Design review of the part built by this model. Coordinates are the model's own, in mm. A direction names the side the tool comes from. Coordinates: 2 decimals unless noted, no trailing zeros. Write each loop counter-clockwise with the first axis right and the second up, starting at its lowest first coordinate (ties: lowest second). Pieces come first, ordered by that corner, then holes.
Q1. For pin 1 Ø1.9 at (x, y) = (5, 25.5) entering from -Z; pin 2 Ø5 at (x, y) = (-20.5, 15.5) entering from -Z; pin 3 Ø2 at (x, z) = (-23.5, 6) entering from +Y, all flat-tipped, find the tip position at first contact; note any pin that passes through.
Q2. For L1, parallel to Y at x = 8, z = 8; L2, parallel to Y at x = 18, z = 6.5 (3 decimals); L3, parallel to X at y = -3.5, z = -2, list the stretches that pass through material, from the lowest coordinate up.
Q3. For faces 1 (the cylindrical face through (-10.211, -24.914, 3.964)), 2 (the flat face through (0.635, 22, 3)), list the 3-axis set-ups (+Z, -Z, +X, -X, +Y, -Y) from which the entire face can be reached by the end or side of a thin tool; tool diameter is ignored.
Q4. The part is to be moulded in two halves that separate along X. For faces 3 (the flat face through (-15.4, -16.3, 2.8)), 4 (the flat face through (28, 0, 11.176)), say which applies: released by +X, released by -X, zero draft, split by the parting line, or undercut.
Q5. Take a section at A-A, the plane z = -6. Write out the cut boundary in (x, y), plus the area to 3 significant figures.
from build123d import *

# Parameters (mm, degrees)
C3A_CAVITYPRISM_DEPTH  = 11.938
SK_C3_RIBS_W           = 19.05
SK_C3_RIBS_H           = 1.27
SK_C3_RIBS_W_2         = 1.27
SK_C3_RIBS_H_2         = 19.05
C3D_RIBS_DEPTH         = 11.938
C2_SCALLOPS_DEPTH      = 47.436868801
C2_SCALLOPS_DEPTH_BACK = 47.436868801
SK_C2_SCALLOPS_R       = 8.382
SK_C5_RIDGE_W          = 3.0426914
SK_C5_RIDGE_H          = 0.381


with BuildPart() as part:
    # SK_C1_profile → C1_MainRevolve (revolve)
    with BuildSketch(Plane(origin=(0, 0, 0), x_dir=(1, 0, 0), z_dir=(0, 1, 0)), mode=Mode.PRIVATE) as c1_mainrevolve_sk:
        with BuildLine():
            Line((0, 17.272), (15.3929334, 17.272))
            ThreePointArc((15.3929334, 17.272), (15.742617524, 17.13249018), (15.900237204, 16.790586666))
            Line((15.900237204, 16.790586666), (16.620448253, 3.048))
            Line((16.620448253, 3.048), (30.48, 3.048))
            Line((30.48, 3.048), (30.48, -11.176))
            Line((30.48, -11.176), (26.924, -11.176))
            ThreePointArc((26.924, -11.176), (19.874523429, -13.957256168), (12.5108462, -15.748))
            Line((12.5108462, -15.748), (0, -15.748))
            Line((0, -15.748), (0, 17.272))
        make_face()
    revolve(c1_mainrevolve_sk.sketch.rotate(Axis((0, 0, -50.8), (0, 0, 1)), 180), axis=Axis((0, 0, -50.8), (0, 0, 1)))

    # SK_C3_Lci → C3a_CavityPrism (cut)
    with BuildSketch(Plane.XY.offset(-3.048)):
        with BuildLine():
            ThreePointArc((27.769715286, -4.872837874), (28.194, 0), (27.769715286, 4.872837874))
            ThreePointArc((27.769715286, 4.872837874), (23.466540126, 9.720159182), (23.081770695, 16.190537286))
            ThreePointArc((23.081770695, 16.190537286), (19.936168589, 19.936168589), (16.190537286, 23.081770695))
            ThreePointArc((16.190537286, 23.081770695), (9.720159182, 23.466540126), (4.872837874, 27.769715286))
            ThreePointArc((4.872837874, 27.769715286), (0, 28.194), (-4.872837874, 27.769715286))
            ThreePointArc((-4.872837874, 27.769715286), (-9.720159182, 23.466540126), (-16.190537286, 23.081770695))
            ThreePointArc((-16.190537286, 23.081770695), (-19.936168589, 19.936168589), (-23.081770695, 16.190537286))
            ThreePointArc((-23.081770695, 16.190537286), (-23.466540126, 9.720159182), (-27.769715286, 4.872837874))
            ThreePointArc((-27.769715286, 4.872837874), (-28.194, 0), (-27.769715286, -4.872837874))
            ThreePointArc((-27.769715286, -4.872837874), (-23.466540126, -9.720159182), (-23.081770695, -16.190537286))
            ThreePointArc((-23.081770695, -16.190537286), (-19.936168589, -19.936168589), (-16.190537286, -23.081770695))
            ThreePointArc((-16.190537286, -23.081770695), (-9.720159182, -23.466540126), (-4.872837874, -27.769715286))
            ThreePointArc((-4.872837874, -27.769715286), (0, -28.194), (4.872837874, -27.769715286))
            ThreePointArc((4.872837874, -27.769715286), (9.720159182, -23.466540126), (16.190537286, -23.081770695))
            ThreePointArc((16.190537286, -23.081770695), (19.936168589, -19.936168589), (23.081770695, -16.190537286))
            ThreePointArc((23.081770695, -16.190537286), (23.466540126, -9.720159182), (27.769715286, -4.872837874))
        make_face()
    extrude(amount=C3A_CAVITYPRISM_DEPTH, mode=Mode.SUBTRACT)


with BuildPart() as c3a_cavityprism_piece_1:
    # of the separate pieces the step leaves, piece 1, a body of its own (c3a_cavityprism_pieces)
    add(part.part.solids().sort_by_distance((-30.48, 0, -3.048))[0])

    # SK_C3_ceiling → C3b_CeilingRing (revolve)
    with BuildSketch(Plane(origin=(0, 0, 0), x_dir=(1, 0, 0), z_dir=(0, 1, 0)), mode=Mode.PRIVATE) as c3b_ceilingring_sk:
        Polygon((25.654, -6.604), (23.368, -8.89), (30.48, -8.89), (30.48, -6.604), align=None)
    revolve(c3b_ceilingring_sk.sketch.rotate(Axis((0, 0, -50.8), (0, 0, 1)), 180), axis=Axis((0, 0, -50.8), (0, 0, 1)))



with BuildPart() as c3a_cavityprism_piece_2:
    # of the separate pieces the step leaves, piece 2, a body of its own (c3a_cavityprism_pieces)
    add(part.part.solids().sort_by_distance((-15.3929334, 0, -17.272))[0])


with BuildPart() as c3a_cavityprism_piece_1_1:
    add(c3a_cavityprism_piece_1.part)

    add(c3a_cavityprism_piece_2.part)  # C3c_HubUp merges C3a_CavityPrism piece 2
    # SK_C3_hub → C3c_HubUp (revolve)
    with BuildSketch(Plane(origin=(0, 0, 0), x_dir=(1, 0, 0), z_dir=(0, 1, 0)), mode=Mode.PRIVATE) as c3c_hubup_sk:
        Polygon((0, 3.048), (16.620448253, 3.048), (17.246092322, -8.89), (0, -8.89), align=None)
    revolve(c3c_hubup_sk.sketch.rotate(Axis((0, 0, -50.8), (0, 0, 1)), 180), axis=Axis((0, 0, -50.8), (0, 0, 1)))

    # SK_C3_ribs → C3d_Ribs (add)
    with BuildSketch(Plane.XY.offset(-3.048)):
        with Locations((19.685, 0)):
            Rectangle(SK_C3_RIBS_W, SK_C3_RIBS_H)
        Polygon((7.633217703, 6.735192091), (21.103601885, 20.205576272), (20.205576272, 21.103601885), (6.735192091, 7.633217703), align=None)
        with Locations((0, 19.685)):
            Rectangle(SK_C3_RIBS_W_2, SK_C3_RIBS_H_2)
        Polygon((-6.735192091, 7.633217703), (-20.205576272, 21.103601885), (-21.103601885, 20.205576272), (-7.633217703, 6.735192091), align=None)
        with Locations((-19.685, 0)):
            Rectangle(SK_C3_RIBS_W, SK_C3_RIBS_H)
        Polygon((-7.633217703, -6.735192091), (-21.103601885, -20.205576272), (-20.205576272, -21.103601885), (-6.735192091, -7.633217703), align=None)
        with Locations((0, -19.685)):
            Rectangle(SK_C3_RIBS_W_2, SK_C3_RIBS_H_2)
        Polygon((6.735192091, -7.633217703), (20.205576272, -21.103601885), (21.103601885, -20.205576272), (7.633217703, -6.735192091), align=None)
    extrude(amount=C3D_RIBS_DEPTH)

    # SK_C2_scallops → C2_Scallops (cut, two sides: drawn at the far end of the back side and taken through both)
    with BuildSketch(Plane.XY.offset(-C2_SCALLOPS_DEPTH_BACK)):
        with Locations((32.618490775, 13.511021263)):
            Circle(SK_C2_SCALLOPS_R)
        with Locations((13.511021263, 32.618490775)):
            Circle(SK_C2_SCALLOPS_R)
        with Locations((-13.511021263, 32.618490775)):
            Circle(SK_C2_SCALLOPS_R)
        with Locations((-32.618490775, 13.511021263)):
            Circle(SK_C2_SCALLOPS_R)
        with Locations((-32.618490775, -13.511021263)):
            Circle(SK_C2_SCALLOPS_R)
        with Locations((-13.511021263, -32.618490775)):
            Circle(SK_C2_SCALLOPS_R)
        with Locations((13.511021263, -32.618490775)):
            Circle(SK_C2_SCALLOPS_R)
        with Locations((32.618490775, -13.511021263)):
            Circle(SK_C2_SCALLOPS_R)
    extrude(amount=C2_SCALLOPS_DEPTH + C2_SCALLOPS_DEPTH_BACK, mode=Mode.SUBTRACT)

    # SK_C4_bore → C4_Bore (revolve, cut)
    with BuildSketch(Plane(origin=(0, 0, 0), x_dir=(1, 0, 0), z_dir=(0, 1, 0)), mode=Mode.PRIVATE) as c4_bore_sk:
        with BuildLine():
            Line((0, 18.542), (6.746875, 18.542))
            Line((6.746875, 18.542), (6.746875, 4.572))
            Line((6.746875, 4.572), (9.144, 4.572))
            Line((9.144, 4.572), (10.1900228, -15.386939))
            ThreePointArc((10.1900228, -15.386939), (10.308227792, -15.643369045), (10.5704894, -15.748))
            Line((10.5704894, -15.748), (10.5704894, -18.288))
            Line((10.5704894, -18.288), (0, -18.288))
            Line((0, -18.288), (0, 18.542))
        make_face()
    revolve(c4_bore_sk.sketch.rotate(Axis((0, 0, -50.8), (0, 0, 1)), 180), axis=Axis((0, 0, -50.8), (0, 0, 1)), mode=Mode.SUBTRACT)

    # SK_C5_ridge → C5_Ridge (revolve)
    with BuildSketch(Plane(origin=(0, 0, 0), x_dir=(1, 0, 0), z_dir=(0, 1, 0)), mode=Mode.PRIVATE) as c5_ridge_sk:
        with Locations((11.3109375, 17.4625)):
            Rectangle(SK_C5_RIDGE_W, SK_C5_RIDGE_H)
    revolve(c5_ridge_sk.sketch.rotate(Axis((0, 0, -50.8), (0, 0, 1)), 180), axis=Axis((0, 0, -50.8), (0, 0, 1)))


solid = c3a_cavityprism_piece_1_1.part
Responses:
1. pin 1: stops at z = 6.6
1. pin 2: stops at z = -3.05
1. pin 3: stops at y = 20.56
2. L1: y = -26.3 to -22.9, -15.23 to -5.67, 5.67 to 15.23, 22.9 to 26.3
2. L2: y = -24.597 to -21.7, -18.898 to -17.102, -0.635 to 0.635, 17.102 to 18.898, 21.7 to 24.597
2. L3: x = -30.28 to -27.98, -16.3 to -8.59, 8.59 to 16.3, 27.98 to 30.28
3. face 1: +Z, -Z, -Y
3. face 2: -Z
4. face 3: undercut
4. face 4: zero draft
5. outline: circle Ø32.93 at (0, 0); hole circle Ø13.49 at (0, 0)
5. area: 709 mm2
